```python
from build123d import *

# Parameters (mm, degrees)
SKETCH_R  = 2.5
PAD_DEPTH = 4.2
FILLET_R  = 1.3


with BuildPart() as part:
    # Sketch → Pad (new body)
    with BuildSketch(Plane.XY):
        with BuildLine():
            Line((-3.9, 0.9), (-3.9, -0.9))
            ThreePointArc((-3.9, -0.9), (-3.02132, -3.02132), (-0.9, -3.9))
            Line((-0.9, -3.9), (0.9, -3.9))
            ThreePointArc((0.9, -3.9), (3.02132, -3.02132), (3.9, -0.9))
            Line((3.9, -0.9), (3.9, 0.9))
            ThreePointArc((3.9, 0.9), (3.02132, 3.02132), (0.9, 3.9))
            Line((0.9, 3.9), (-0.9, 3.9))
            ThreePointArc((-0.9, 3.9), (-3.02132, 3.02132), (-3.9, 0.9))
        make_face()
        Circle(SKETCH_R, mode=Mode.SUBTRACT)
    extrude(amount=PAD_DEPTH)

    # Fillet
    fillet_edges = [part.edges().sort_by_distance(p)[0] for p in [
        (3.9, 0, 4.2),
    ]]
    fillet(fillet_edges, radius=FILLET_R)


solid = part.part
```
The listing builds one solid part. Answer for the finished solid, in the listing's coordinates (mm). Coordinates: 2 decimals unless noted, no trailing zeros. Loops run counter-clockwise (first coordinate to the right, second up) from the corner with the lowest first, then second, coordinate; pieces in that order, holes last. Notation, with made-up numbers: M -5.5,3.25 L 26.5,3.25 A15 ccw 26.5,9.25 Z; hole C -17,-1 d9. An arc over 180 degrees is marked long. Answer as a JSON object with one key per item and string values. Group by question number.
Item 1: Section A-A (y = 0) is taken. Write down the section's boundary in (x, z), and give its area (3 significant figures).
Item 2: Determine the mould class of faces 1 (the face through (-0.01, 3.53, 3.81)), 2 (the face through (-0.54, -2.44, 2.07)), 3 (the face through (0, -3.9, 1)), 4 (the face through (-3.53, -0.01, 3.81)) for opening direction Y: +Y half, -Y half, draft (parallel to the pull), parting line (faces both ways), or undercut.
Item 3: Consider L1, parallel to Y at x = 0, z = 1.55; L2, parallel to X at y = 0.25, z = 1.3; L3, parallel to Y at x = 0.75, z = 1.35. Determine where each line is inside the solid, lowest interval first.
Item 4: Section D-D (z = 3.7) is taken. Write down the section's boundary in (x, y).
Item 5: Section C-C (z = 1.8) is taken. Write down the section's boundary in (x, y).
Solved:
{
 "1": {"outline": "M -3.9,0 L -2.5,0 L -2.5,4.2 L -2.6,4.2 A1.3 ccw -3.9,2.9 Z; M 2.5,0 L 3.9,0 L 3.9,2.9 A1.3 ccw 2.6,4.2 L 2.5,4.2 Z", "area": "11.0 mm2"},
 "2": {"face 1": "+Y half", "face 2": "undercut", "face 3": "-Y half", "face 4": "draft"},
 "3": {"L1": "y = -3.9 to -2.5, 2.5 to 3.9", "L2": "x = -3.9 to -2.49, 2.49 to 3.9", "L3": "y = -3.9 to -2.38, 2.38 to 3.9"},
 "4": {"outline": "M -3.62,-0.9 A2.72 ccw -0.9,-3.62 L 0.9,-3.62 A2.72 ccw 3.62,-0.9 L 3.62,0.9 A2.72 ccw 0.9,3.62 L -0.9,3.62 A2.72 ccw -3.62,0.9 Z; hole C 0,0 d5"},
 "5": {"outline": "M -3.9,-0.9 A3 ccw -0.9,-3.9 L 0.9,-3.9 A3 ccw 3.9,-0.9 L 3.9,0.9 A3 ccw 0.9,3.9 L -0.9,3.9 A3 ccw -3.9,0.9 Z; hole C 0,0 d5"}
}
